Input: part model. Units: mm. Frame: model coordinates. Face numbers are marked on the shaded views. Coordinates: 2 decimals unless noted, no trailing zeros. Write each loop counter-clockwise with the first axis right and the second up, starting at its lowest first coordinate (ties: lowest second). Pieces come first, ordered by that corner, then holes. Notation, with made-up numbers: (53, 79.5) -> (107, 79.5) arc R12 cw to (107, 93.5) -> close; hole circle Ø2 at (77.25, 46). An arc over 180 degrees is marked (long way). Use one line per item in the form item = value. Start each with the question number.
(1) Cut plane A-A on x = 0. Return the cut outline in (y, z), plus the area to 3 significant figures.
(2) Cut plane D-D on y = 5. Return the cut outline in (x, z), plus the area to 3 significant figures.
(3) Cut plane C-C on z = 1.5. Return the cut outline in (x, y).
(4) Ray query, line 1 along X through (y, z) = (0, -0.95); line 2 along Y through (x, z) = (0, -1.05); line 3 along Y through (x, z) = (1, -0.4). Return the intervals inside material, ascending.
(5) Cut plane B-B on y = -1. Return the cut outline in (x, z), plus the area to 3 significant figures.
(6) First-contact query: pin 1 (1 mm diameter, centred on x = -0.5, z = 2, fed in from +Y). Flat tip, straight axial feed; report the tip coordinate or a pass-through.
(7) Pull-direction query (Y, two-part tool) for the marked faces 1, 2 and 3; classes: released by +Y, released by -Y, zero draft, split by the parting line, or undercut.
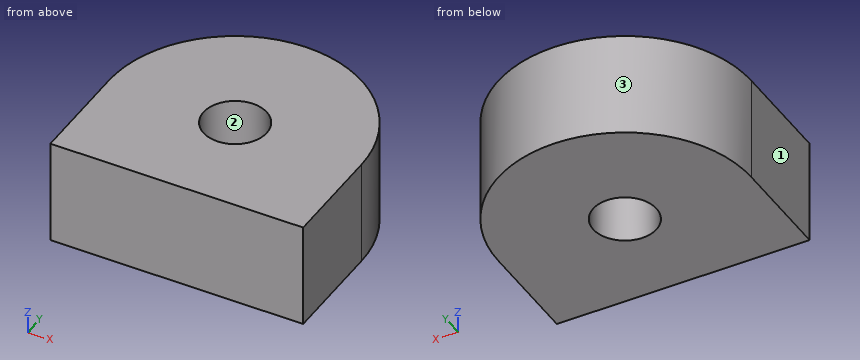
```python
from build123d import *

# Parameters (mm, degrees)
BOSS_EXTRUDE1_DEPTH     = 2.5
SKETCH4_R               = 1.5
CUT_EXTRUDE1_DEPTH      = 3.5
CUT_EXTRUDE1_DEPTH_BACK = 3.5


with BuildPart() as part:
    # Sketch2 → Boss-Extrude1 (new body, symmetric)
    with BuildSketch(Plane.XY):
        with BuildLine():
            Line((-6, 0), (-6, -5))
            Line((-6, -5), (6, -5))
            Line((6, -5), (6, 0))
            ThreePointArc((6, 0), (0, 6), (-6, 0))
        make_face()
    extrude(amount=BOSS_EXTRUDE1_DEPTH, both=True)

    # Sketch4 → Cut-Extrude1 (cut, two sides)
    with BuildSketch(Plane.XY) as cut_extrude1_sk:
        Circle(SKETCH4_R)
    extrude(amount=CUT_EXTRUDE1_DEPTH, mode=Mode.SUBTRACT)
    extrude(cut_extrude1_sk.sketch, amount=-CUT_EXTRUDE1_DEPTH_BACK, mode=Mode.SUBTRACT)


solid = part.part
```
Values:
q1.outline = (-5, -2.5) -> (-1.5, -2.5) -> (-1.5, 2.5) -> (-5, 2.5) -> close; (1.5, -2.5) -> (6, -2.5) -> (6, 2.5) -> (1.5, 2.5) -> close
q1.area = 40.0 mm2
q2.outline = (-3.32, -2.5) -> (3.32, -2.5) -> (3.32, 2.5) -> (-3.32, 2.5) -> close
q2.area = 33.2 mm2
q3.outline = (-6, -5) -> (6, -5) -> (6, 0) arc R6 ccw to (-6, 0) -> close; hole circle Ø3 at (0, 0)
q4.line_1 = -6 to -1.5, 1.5 to 6
q4.line_2 = -5 to -1.5, 1.5 to 6
q4.line_3 = -5 to -1.12, 1.12 to 5.92
q5.outline = (-6, -2.5) -> (-1.12, -2.5) -> (-1.12, 2.5) -> (-6, 2.5) -> close; (1.12, -2.5) -> (6, -2.5) -> (6, 2.5) -> (1.12, 2.5) -> close
q5.area = 48.8 mm2
q6.pin_1 = 6
q7.face_1 = zero draft
q7.face_2 = undercut
q7.face_3 = released by +Y
